```python
from build123d import *

# Parameters (mm, degrees)
F1_W      = 10
F1_H      = 10
F1_W_2    = 6
F1_H_2    = 6
F5_W      = 10
F5_H      = 10
F5_W_2    = 6
F5_H_2    = 6
F8_DEPTH  = 3
F10_COUNT = 6


with BuildPart() as f2:
    # F2: sweep along a path in F0
    with BuildLine(Plane.XZ) as f2_path:
        Line((-37.5, 64.9519052838), (37.5, 64.9519052838))
        Line((37.5, 64.9519052838), (75, 0))
        Line((75, 0), (37.5, -64.9519052838))
        Line((37.5, -64.9519052838), (-37.5, -64.9519052838))
        Line((-37.5, -64.9519052838), (-75, 0))
        Line((-75, 0), (-37.5, 64.9519052838))
    # F1 (on Right) → F2 (sweep)
    with BuildSketch(Plane.YZ):
        with Locations((0, 64.9519052838)):
            Rectangle(F1_W, F1_H)
        with Locations((0, 64.9519052838)):
            Rectangle(F1_W_2, F1_H_2, mode=Mode.SUBTRACT)
    sweep(path=f2_path.line, transition=Transition.RIGHT)



with BuildPart() as f6:
    # F6: sweep along a path in F4
    with BuildLine(Plane.XZ.offset(35)) as f6_path:
        Line((17.5, -30.3108891325), (-17.5, -30.3108891325))
        Line((-17.5, -30.3108891325), (-35, 0))
        Line((-35, 0), (-17.5, 30.3108891325))
        Line((-17.5, 30.3108891325), (17.5, 30.3108891325))
        Line((17.5, 30.3108891325), (35, 0))
        Line((35, 0), (17.5, -30.3108891325))
    # F5 (on Right) → F6 (sweep)
    with BuildSketch(Plane.YZ):
        with Locations((-35, -30.3108891325)):
            Rectangle(F5_W, F5_H)
        with Locations((-35, -30.3108891325)):
            Rectangle(F5_W_2, F5_H_2, mode=Mode.SUBTRACT)
    sweep(path=f6_path.line, transition=Transition.RIGHT)


with BuildPart() as f2_1:
    add(f2.part)

    add(f6.part)  # F8 merges F6
    # F7 (on Top) → F8 (join, symmetric)
    with BuildSketch(Plane.XY):
        Polygon((71.7735026919, -5), (32.2735026919, -30), (38.2735026919, -30), (77.7735026919, -5), align=None)
    extrude(amount=F8_DEPTH, both=True)

    # F10: F2 ×6 about axis
    f10_axis = Axis((0, -16.170989722, 0), (0, 1, 0))


with BuildPart() as f2_2:
    add(f2_1.part)
    for i in range(1, F10_COUNT):
        add(f2_1.part.rotate(f10_axis, i * 360 / F10_COUNT))


solid = f2_2.part
```
Can you work these out from the model? Positions are in its coordinate system, mm. A direction names the side the tool comes from. Coordinates: 2 decimals unless noted, no trailing zeros. Loops run counter-clockwise (first coordinate to the right, second up) from the corner with the lowest first, then second, coordinate; pieces in that order, holes last.
1) Thinking about a two-plate mould opening in X: for faces 6 (the flat face through (30.44, -35.07, -17.9)), 7 (the flat face through (23.54, -35.04, -13.85)), 8 (the flat face through (53.4, 0.04, -31.41)), 9 (the flat face through (-30.057, -17.442, 46.06)), which applies, pulls with the +X half, pulls with the -X half, needs draft (parallel to the pull), parting line crosses it, or undercut?
2) Imagine slicing it at B-B on z = -41. List the corners of the cut face in (x, y) for me, plus the area to 3 significant figures.
3) Imagine slicing it at A-A on y = 1. List the corners of the cut face in (x, z) for me.
4) For pin 1 (8 mm diameter, centred on x = 7, y = -36.5, fed in from +Z); pin 2 (7.5 mm diameter, centred on x = -51.5, y = -23.5, fed in from -Z); pin 3 (1 mm diameter, centred on y = -12, z = 0, fed in from +X), each with a flat end and sliding along its axis, tell me the tip position at first contact or that it passes through.
5) I need wall thicknesses on probe 1 along Z at (x, y) = (-11.5, -35); probe 2 along Y at (x, z) = (-67.5, -10.5); probe 3 along X at (y, z) = (0.5, -61.5). Which ranges of each line are inside material? Lowest first, please.
6) Imagine slicing it at D-D on x = 50.5. List the corners of the cut face in (y, z) for me.
7) Imagine slicing it at C-C on x = -6.5. State how many separate pieces and enclosed holes the cut face has, plus the area to 3 significant figures.
8) Which directions (+Z, -Z, +X, -X, +Y, -Y) give clear straight access to the entire face, cutting with the end or side of a thin tool? Please do faces 1 (the flat face through (-58.573, -0.042, 34.452)), 2 (the flat face through (-59, 5, 20)), 3 (the flat face through (21.82, -34.93, -12.83)), 4 (the flat face through (0, -35, 35.311)), 5 (the flat face through (60.297, 0.07, -35.466)).
Completed:
1. face 6: pulls with the +X half
1. face 7: undercut
1. face 8: undercut
1. face 9: pulls with the -X half
2. outline: (-57.1, -5) - (-45.56, -5) - (-45.56, 5) - (-57.1, 5) - close; (-27.14, -23.16) - (-20.21, -25.36) - (-20.21, -21.56) - (-27.14, -19.37) - close; (20.21, -25.36) - (27.14, -23.16) - (27.14, -19.37) - (20.21, -21.56) - close; (45.56, -5) - (57.1, -5) - (57.1, 5) - (45.56, 5) - close; hole (-54.79, -3) - (-47.86, -3) - (-47.86, 3) - (-54.79, 3) - close; hole (47.86, -3) - (54.79, -3) - (54.79, 3) - (47.86, 3) - close
2. area: 200 mm2
3. outline: (-80.77, 0) - (-40.39, -69.95) - (40.39, -69.95) - (80.77, 0) - (40.39, 69.95) - (-40.39, 69.95) - close; (-71.54, 0) - (-35.77, -61.95) - (35.77, -61.95) - (71.54, 0) - (35.77, 61.95) - (-35.77, 61.95) - close; hole (-78.46, 0) - (-39.23, -67.95) - (39.23, -67.95) - (78.46, 0) - (39.23, 67.95) - (-39.23, 67.95) - close; hole (-69.23, 0) - (-34.61, -59.95) - (34.61, -59.95) - (69.23, 0) - (34.61, 59.95) - (-34.61, 59.95) - close
4. pin 1: stops at z = 35.31
4. pin 2: stops at z = -3
4. pin 3: stops at x = 67.5
5. probe 1: z = -35.31 to -33.31, -27.31 to -25.31, 25.31 to 27.31, 33.31 to 35.31
5. probe 2: y = -5 to -3, 3 to 5
5. probe 3: x = -45.27 to -42.96, -36.03 to 36.03, 42.96 to 45.27
6. outline: (-22.26, -3) - (-18.46, -3) - (-18.46, 3) - (-22.26, 3) - close; (-5, -52.44) - (5, -52.44) - (5, -32.44) - (-5, -32.44) - close; (-5, 32.44) - (5, 32.44) - (5, 52.44) - (-5, 52.44) - close; hole (-3, -48.44) - (3, -48.44) - (3, -36.44) - (-3, -36.44) - close; hole (-3, 36.44) - (3, 36.44) - (3, 48.44) - (-3, 48.44) - close
7. separate pieces: 4
7. enclosed holes: 4
7. area: 256 mm2
8. face 1: none
8. face 2: +Z, -Z, +X, -X, +Y
8. face 3: +Y, -Y
8. face 4: +Z, +X, -X, -Y
8. face 5: -Z, +X, +Y, -Y
